Could you check a few things on this model? Use its own coordinates, in mm. A direction names the side the tool comes from. Round coordinates to 2 decimals unless told otherwise and drop trailing zeros. Loops run counter-clockwise (first coordinate to the right, second up) from the corner with the lowest first, then second, coordinate; pieces in that order, holes last. Notation, with made-up numbers: M 32,-14.75 L 40,-14.75 A23 ccw 40,20.25 Z; hole C 21,48 d11. An arc over 180 degrees is marked long. Answer in a Markdown table with one row per item.
```python
from build123d import *

# Parameters (mm, degrees)
SKETCH1_W           = 35
SKETCH1_H           = 9.4
BOSS_EXTRUDE1_DEPTH = 2.8
SKETCH2_W           = 3.1
SKETCH2_H           = 1.6
CUT_EXTRUDE1_DEPTH  = 35
CHAMFER2_SIZE       = 4
CHAMFER5_SIZE       = 1
CHAMFER5_SIZE2      = 0.577350269
CHAMFER6_SIZE       = 1
CHAMFER6_SIZE2      = 0.577350269
CUT_EXTRUDE2_DEPTH  = 10


with BuildPart() as part:
    # Sketch1 → Boss-Extrude1 (new body)
    # profile 1 of 2: a face of its own
    with BuildSketch(Plane(origin=(0, 0, 0), x_dir=(1, 0, 0), z_dir=(0, 1, 0))):
        with Locations((17.5, 4.7)):
            Rectangle(SKETCH1_W, SKETCH1_H)
    # profile 2 of 2: a face of its own
    with BuildSketch(Plane(origin=(0, 0, 0), x_dir=(1, 0, 0), z_dir=(0, 1, 0))):
        Polygon((35, 0), (35, 9.4), (43.140638796, 14.1), (51.281277591, 9.4), (51.281277591, 0), (43.140638796, -4.7), align=None)
        with BuildLine():
            ThreePointArc((45.140638796, 2.2), (46.640638796, 0.7), (48.140638796, 2.2))
            Line((48.140638796, 2.2), (48.140638796, 7.2))
            ThreePointArc((48.140638796, 7.2), (46.640638796, 8.7), (45.140638796, 7.2))
            Line((45.140638796, 7.2), (45.140638796, 2.2))
        make_face(mode=Mode.SUBTRACT)
    extrude(amount=BOSS_EXTRUDE1_DEPTH)

    # Sketch2 → Cut-Extrude1 (cut)
    with BuildSketch(Plane.ZY):
        with Locations((-4.45, 0.8)):
            Rectangle(SKETCH2_W, SKETCH2_H)
    extrude(amount=-CUT_EXTRUDE1_DEPTH, mode=Mode.SUBTRACT)

    # Chamfer2
    chamfer2_edges = [part.edges().sort_by_distance(p)[0] for p in [
        (0, 1.4, 0),
    ]]
    chamfer(chamfer2_edges, length=CHAMFER2_SIZE)

    # Chamfer5
    chamfer5_edges = [part.edges().sort_by_distance(p)[0] for p in [
        (19.5, 0, 0),
    ]]
    chamfer5_side = [part.faces().sort_by_distance(p)[0] for p in [
        (18.05, 0, -2.353812355),
    ]]
    chamfer(chamfer5_edges, length=CHAMFER5_SIZE, length2=CHAMFER5_SIZE2, reference=chamfer5_side[0])

    # Chamfer6
    chamfer6_edges = [part.edges().sort_by_distance(p)[0] for p in [
        (19.5, 2.8, 0),
    ]]
    chamfer6_side = [part.faces().sort_by_distance(p)[0] for p in [
        (27.665536573, 2.8, -4.750962089),
    ]]
    chamfer(chamfer6_edges, length=CHAMFER6_SIZE, length2=CHAMFER6_SIZE2, reference=chamfer6_side[0])

    # Sketch3 → Cut-Extrude2 (cut)
    with BuildSketch(Plane(origin=(0, 2.8, 0), x_dir=(1, 0, 0), z_dir=(0, 1, 0))):
        Polygon((8, 8.4), (10.5, 8.4), (13.5, 7.4), (16, 7.4), (18.5, 7.4), (21.5, 7.9), (24, 7.9), (26.5, 7.9), (28, 9.4), (4, 9.4), (0, 9.4), (0, 5.4), (5.5, 8.4), align=None)
    extrude(amount=-CUT_EXTRUDE2_DEPTH, mode=Mode.SUBTRACT)


solid = part.part
```
1) Will these pins go through, and if not, where does the flat tip stop? P1, Ø1.4, axis at x = 7, y = 1.5, coming from the -Z side; P2, Ø1.5, axis at x = 25, z = -4.5, coming from the -Y side; P3, Ø6, axis at x = 39, z = -7, coming from the -Y side; P4, Ø0.8, axis at x = 23, y = 2, coming from the -Z side.
Computed:
| item | result |
|---|---|
| P1 | stops at z = -8.4 |
| P2 | stops at y = 1.6 |
| P3 | stops at y = 0 |
| P4 | stops at z = -7.9 |
2) I want a section at B-B, the plane z = -1.75. Please give me the cut outline in (x, y).
Computed:
| item | result |
|---|---|
| outline | M 2.25,0 L 45.21,0 L 45.21,2.8 L 2.25,2.8 Z; M 48.07,0 L 51.28,0 L 51.28,2.8 L 48.07,2.8 Z |
3) I want a section at A-A, the plane x = 12. Please give me the cut outline in (y, z), plus the area to 3 significant figures.
Computed:
| item | result |
|---|---|
| outline | M 0,-7.9 L 2.8,-7.9 L 2.8,-1 L 2.22,0 L 0.58,0 L 0,-1 L 0,-2.9 L 1.6,-2.9 L 1.6,-6 L 0,-6 Z |
| area | 16.6 mm² |
4) Which directions (+Z, -Z, +X, -X, +Y, -Y) give clear straight access to the entire face, cutting with the end or side of a thin tool? Please do faces 1 (the face through (32, 2.8, -5)), 2 (the face through (19.979, 1.42, -7.647)), 3 (the face through (35, 1, -4)), 4 (the face through (45.141, 1, -5)), 5 (the face through (31, 1, -9.4)).
Computed:
| item | result |
|---|---|
| face 1 | +Z, -Z, +X, -X, +Y |
| face 2 | -Z, +Y, -Y |
| face 3 | -X, -Y |
| face 4 | +Y, -Y |
| face 5 | -Z, -X, +Y, -Y |
5) If we mould it in two halves opening along Z, with no side actions, what happens to faces 6 (the face through (46.6, 1.4, -0.7)), 7 (the face through (51.281, 1, -5)), 8 (the face through (18.776, 2.507, -0.493))? For each: released by +Z, released by -Z, zero draft, split by the parting line, or undercut.
Computed:
| item | result |
|---|---|
| face 6 | undercut |
| face 7 | zero draft |
| face 8 | released by +Z |
6) I need wall thicknesses on line 1 (X direction, y = 1.35, z = -3); line 2 (Z direction, x = 23, y = 1.55); line 3 (Y direction, x = 30, z = -4.25). Which ranges of each line are inside material? Lowest first, please.
Computed:
| item | result |
|---|---|
| line 1 | x = 35 to 45.14, 48.14 to 51.28 |
| line 2 | z = -7.9 to -6, -2.9 to 0 |
| line 3 | y = 1.6 to 2.8 |
7) I want a section at D-D, the plane z = 2.5. Please give me the cut outline in (x, y), plus the area to 3 significant figures.
Computed:
| item | result |
|---|---|
| outline | M 39.33,0 L 46.95,0 L 46.95,2.8 L 39.33,2.8 Z |
| area | 21.3 mm² |
8) I want a section at C-C, the plane x = 31. Please give me the cut outline in (y, z).
Computed:
| item | result |
|---|---|
| outline | M 0,-9.4 L 2.8,-9.4 L 2.8,-1 L 2.22,0 L 0.58,0 L 0,-1 L 0,-2.9 L 1.6,-2.9 L 1.6,-6 L 0,-6 Z |
